Drawing for the job (mm, zero at the part's lowest x, y, z). A direction names the side the tool comes from. Coordinates: 2 decimals unless noted, no trailing zeros. Order: outer loops, then holes, each group sorted by start corner. A loop starts at its lowest first (then second) coordinate and runs counter-clockwise, first axis right, second up. Notation, with made-up numbers: M 5.25,71 L 47.25,71 A21 cw 47.25,96 Z; hole C 82,41 d11. An arc over 180 degrees is marked long. Write item = value, one per line. Start each with the question number.
Q1. 3-axis set-ups, long thin cutter, end or side, ignore diameter. For the marked faces 1 and 2: which of +Z, -Z, +X, -X, +Y, -Y reach the whole face in a straight line?
Q2. Band-saw the part on B-B on x = 22.5. Write the cut outline in (y, z), plus the area to 3 significant figures.
Q3. Band-saw the part on A-A on z = 15. Write the cut outline in (x, y), plus the area to 4 significant figures.
Q4. Drill centre lines: probe 1 along Y at (x, z) = (22.5, 2.75); probe 2 along Z at (x, y) = (17.5, 11.5); probe 3 along Y at (x, z) = (34.5, 7). Where is each one in solid material? Low to high.
Q5. Band-saw the part on C-C on y = 12. Write the cut outline in (x, z).
Q6. Pin check, flat tips, straight feed: P1, Ø8, axis at x = 18, y = 11, coming from the +Z side; P2, Ø9, axis at y = 7, z = 13.5, coming from the +X side; P3, Ø8.5, axis at x = 22.5, y = 16, coming from the -Z side; P4, Ø6, axis at x = 18, z = 15, coming from the -Y side. Stop position of each tip, or through.
Q7. Band-saw the part on D-D on z = 8. Write the cut outline in (x, y).
Q8. Pull direction Z, two halves, no side cores. Call the marked faces 3, 4 and 5: released by +Z, released by -Z, zero draft, split by the parting line, or undercut.
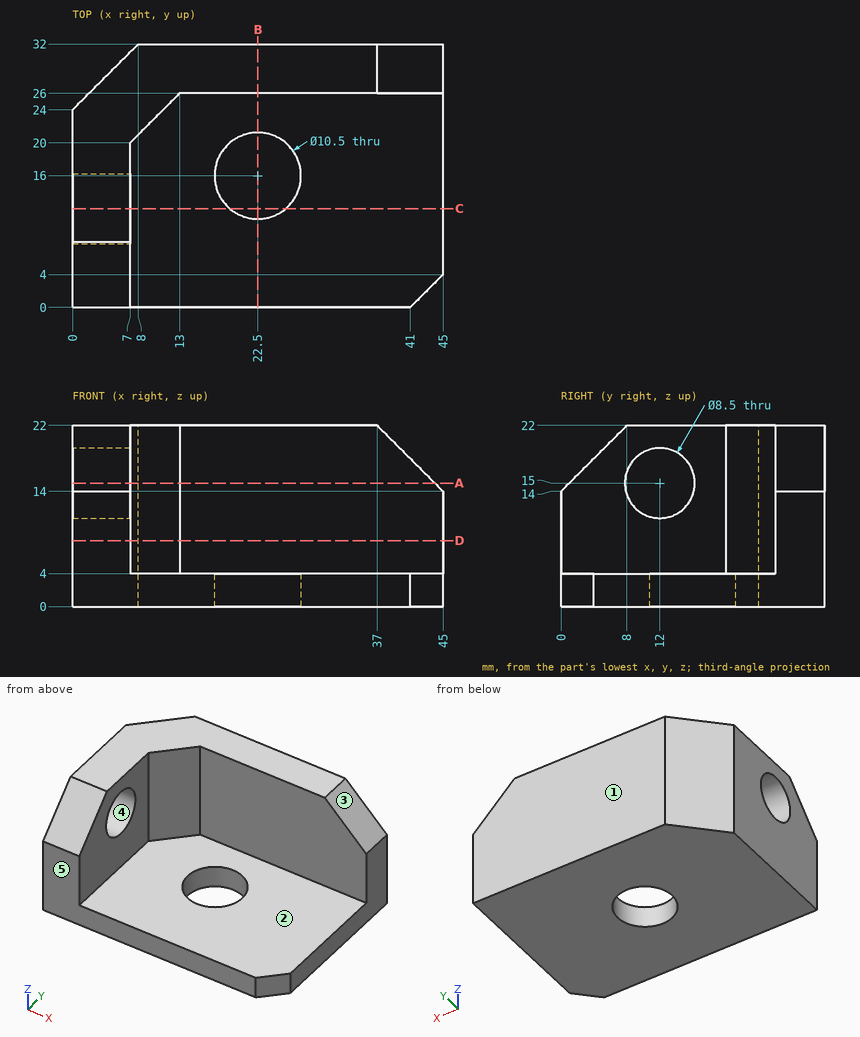
Recorded:
q1.face_1 = +Z, -Z, +X, -X, +Y
q1.face_2 = +Z, +X, -Y
q2.outline = M 0,0 L 10.75,0 L 10.75,4 L 0,4 Z; M 21.25,0 L 32,0 L 32,22 L 26,22 L 26,4 L 21.25,4 Z
q2.area = 194 mm2
q3.outline = M 0,1 L 7,1 L 7,7.75 L 0,7.75 Z; M 0,16.25 L 7,16.25 L 7,20 L 13,26 L 44,26 L 44,32 L 8,32 L 0,24 Z
q3.area = 365.5 mm2
q4.probe_1 = 0 to 10.75, 21.25 to 32
q4.probe_2 = 0 to 4
q4.probe_3 = 26 to 32
q5.outline = M 0,0 L 19.1,0 L 19.1,4 L 7,4 L 7,10.75 L 0,10.75 Z; M 0,19.25 L 7,19.25 L 7,22 L 0,22 Z; M 25.9,0 L 45,0 L 45,4 L 25.9,4 Z
q6.P1 = 4
q6.P2 = 7
q6.P3 = through
q6.P4 = 26
q7.outline = M 0,0 L 7,0 L 7,20 L 13,26 L 45,26 L 45,32 L 8,32 L 0,24 Z
q8.face_3 = released by +Z
q8.face_4 = undercut
q8.face_5 = zero draft
